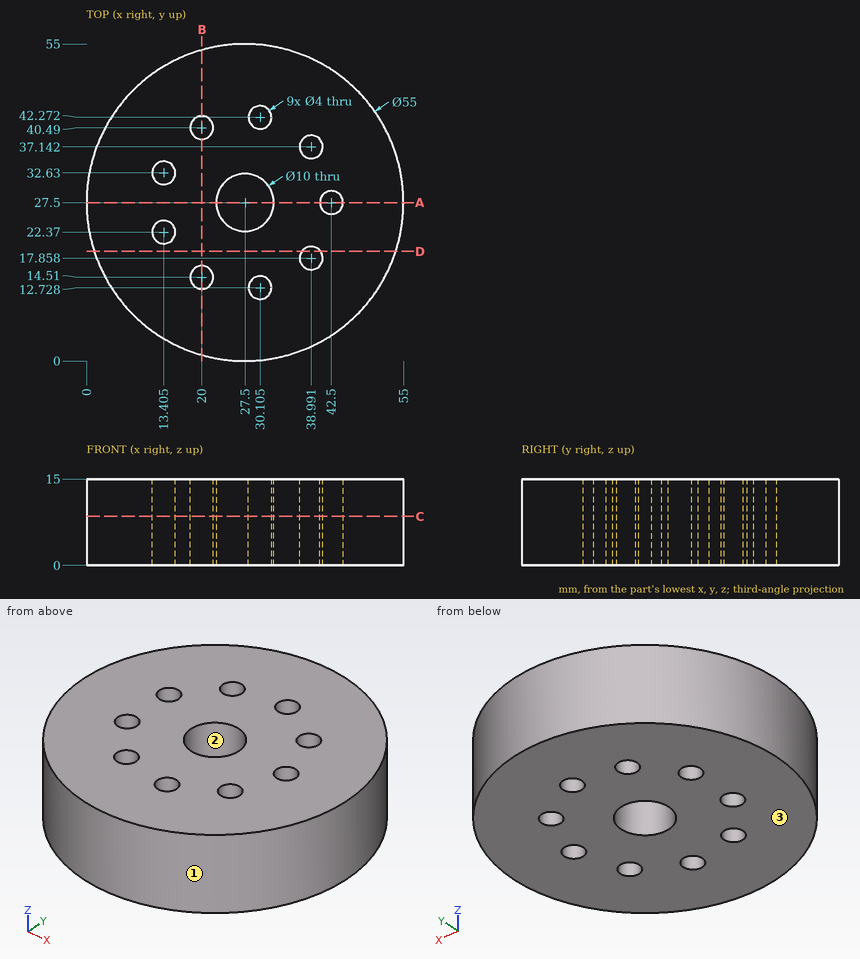
Study the drawing (mm; zero at the part's minimum x, y, z) and answer. Round coordinates to 2 decimals unless told otherwise and drop trailing zeros. Order: outer loops, then holes, each group sorted by start corner. A loop starts at its lowest first (then second) coordinate and runs counter-clockwise, first axis right, second up. Notation, with made-up numbers: (18, 55.5) -> (64, 55.5) arc R20 ccw to (64, 91.5) -> close; hole circle Ø11 at (-6, 17.5). An arc over 180 degrees is marked (long way). Write each question's results on one line, items separated by ' | '. Start each with the question number.
Q1. Find section D-D (y = 19). Determine the outline of the cut face in (x, z), then the cut area to 3 significant figures.
Q2. The mould has two halves that part along X. Classify the marked faces 1, 2 and 3: pulls with the +X half, pulls with the -X half, needs draft (parallel to the pull), parting line crosses it, or undercut.
Q3. Each of these flat-tipped pins is pushed along its axis until it touches: pin 1 (8 mm diameter, centred on y = 17.5, z = 2.5, fed in from -X); pin 2 (8 mm diameter, centred on y = 15, z = 10.5, fed in from +X); pin 3 (8 mm diameter, centred on x = 32, z = 7, fed in from -Y). Where does it stop, or does it pass through?
Q4. Straight lines are drawn through the part: probe 1 along Y at (x, z) = (37.5, 13) (1 decimal); probe 2 along Y at (x, z) = (13.5, 4); probe 3 along X at (y, z) = (17.5, 2.75). For each, find the intervals that lie inside material, in ascending order. Write a range as from..to.
Q5. Find section B-B (x = 20). Determine the outline of the cut face in (y, z), then the cut area to 3 significant figures.
Q6. Find section C-C (z = 8.5). Give the number of separate pieces and of enclosed holes in the cut face, then the cut area to 3 significant figures.
Q7. Find section A-A (y = 27.5). Determine the outline of the cut face in (x, z).
Worked answers:
1) outline: (1.35, 0) -> (37.35, 0) -> (37.35, 15) -> (1.35, 15) -> close; (40.63, 0) -> (53.65, 0) -> (53.65, 15) -> (40.63, 15) -> close | area: 735 mm2
2) face 1: parting line crosses it | face 2: undercut | face 3: needs draft
3) pin 1: stops at x = 0.66 | pin 2: stops at x = 53.65 | pin 3: stops at y = 0
4) probe 1: y = 1.9..16.5, 19.2..35.8, 38.5..53.1 | probe 2: y = 3.83..20.37, 24.37..30.63, 34.63..51.17 | probe 3: x = 1.88..37.02, 40.96..53.12
5) outline: (1.04, 0) -> (12.51, 0) -> (12.51, 15) -> (1.04, 15) -> close; (16.51, 0) -> (38.49, 0) -> (38.49, 15) -> (16.51, 15) -> close; (42.49, 0) -> (53.96, 0) -> (53.96, 15) -> (42.49, 15) -> close | area: 674 mm2
6) separate pieces: 1 | enclosed holes: 10 | area: 2,180 mm2
7) outline: (0, 0) -> (22.5, 0) -> (22.5, 15) -> (0, 15) -> close; (32.5, 0) -> (40.5, 0) -> (40.5, 15) -> (32.5, 15) -> close; (44.5, 0) -> (55, 0) -> (55, 15) -> (44.5, 15) -> close
